Can you work these out from the model? Positions are in its coordinate system, mm. A direction names the side the tool comes from. Round coordinates to 2 decimals unless told otherwise and drop trailing zeros. Loops run counter-clockwise (first coordinate to the right, second up) from the corner with the lowest first, then second, coordinate; pieces in that order, holes last. Notation, with made-up numbers: M -34,0.25 L -27,0.25 A22 cw -27,27.25 Z; hole C 61.5,74.25 d5. An arc over 180 degrees is marked long. Answer as CSV lines item,"result".
from build123d import *

# Parameters (mm, degrees)
SKETCH1_R                                 = 21.166666667
BOSS_EXTRUDE1_DEPTH                       = 12.7
CUT_EXTRUDE_DCLTBC_DEPTH                  = 13.7
FILLET_TIP_DCLTBC_R                       = 0.376401082
FILLET_ROOT_DCLTBC_R                      = 0.752802164
CIRPATTERN_DCLTBC_COUNT                   = 18
FILLET_TIP_DCLTBC_OF_CIRPATTERN_DCLTBC_R  = 0.376401082
FILLET_ROOT_DCLTBC_OF_CIRPATTERN_DCLTBC_R = 0.752802164
SKETCH4_R                                 = 3.556
CUT_EXTRUDE2_DEPTH                        = 13.7000001
SKETCH5_R                                 = 1
CUT_EXTRUDE3_DEPTH                        = 13.7000001
BOSS_EXTRUDE3_DEPTH                       = 12.7
SKETCH9_R                                 = 1.778
CUT_EXTRUDE4_DEPTH                        = 101.6
SKETCH10_R                                = 2.75
CUT_EXTRUDE5_DEPTH                        = 7.7
CUT_EXTRUDE6_DEPTH                        = 13.7000001
CIRPATTERN1_COUNT                         = 30
CIRPATTERN1_ANGLE                         = 75
SKETCH12_W                                = 54.92757211
SKETCH12_H                                = 48.855993121
CUT_EXTRUDE7_DEPTH                        = 13.7000001


with BuildPart() as part:
    # Sketch1 → Boss-Extrude1 (new body)
    with BuildSketch(Plane.XY):
        Circle(SKETCH1_R)
    extrude(amount=BOSS_EXTRUDE1_DEPTH)

    # DCLTBC → Cut-Extrude-DCLTBC (cut, through all)
    with BuildSketch(Plane.XY):
        with BuildLine():
            Line((-0.988599485, 17.23683661), (-0.939299003, 16.37725256))
            ThreePointArc((-0.939299003, 16.37725256), (0, 16.404166667), (0.939299003, 16.37725256))
            Line((0.939299003, 16.37725256), (0.988599485, 17.23683661))
            add(Edge.make_bspline(
                [(0.988599485, 17.23683661), (0.989063314, 17.24324115), (0.990661792, 17.261181979), (0.994858273, 17.295004515), (1.003369641, 17.350013815), (1.016655031, 17.419804647), (1.036619493, 17.509601098), (1.063718234, 17.614795353), (1.097234262, 17.729707804), (1.137709634, 17.85389969), (1.181621422, 17.977005275), (1.228695452, 18.099012466), (1.278527467, 18.219794849), (1.342341331, 18.365146152), (1.42364652, 18.538069209), (1.525589195, 18.738036686), (1.649316002, 18.962165854), (1.783980218, 19.187521629), (1.923498112, 19.406676656), (2.072405817, 19.624910262), (2.222105415, 19.833784741), (2.385586794, 20.047220122), (2.540566559, 20.242458208), (2.722891612, 20.457068476), (2.872582231, 20.629074977), (3.034353491, 20.803165616), (3.114136758, 20.887359483), (3.155350355, 20.930158669)],
                knots=[0, 0, 0, 0, 0, 0.005376749, 0.015083688, 0.02853182, 0.04661014, 0.064854849, 0.092110525, 0.119476176, 0.146842496, 0.174208854, 0.201574956, 0.228941013, 0.256307345, 0.307035032, 0.361767352, 0.416499661, 0.471231937, 0.525964282, 0.580696616, 0.635428982, 0.690161387, 0.744893688, 0.799626082, 0.854358408, 0.909090915, 0.909090915, 0.909090915, 0.909090915, 0.909090915], degree=4))
            ThreePointArc((3.155350355, 20.930158669), (0, 21.166666667), (-3.155350355, 20.930158669))
            add(Edge.make_bspline(
                [(-0.988599485, 17.23683661), (-0.989063314, 17.24324115), (-0.990661792, 17.261181979), (-0.994858273, 17.295004515), (-1.003369641, 17.350013815), (-1.016655031, 17.419804647), (-1.036619493, 17.509601098), (-1.063718234, 17.614795353), (-1.097234262, 17.729707804), (-1.137709634, 17.85389969), (-1.181621422, 17.977005275), (-1.228695452, 18.099012466), (-1.278527467, 18.219794849), (-1.342341331, 18.365146152), (-1.42364652, 18.538069209), (-1.525589195, 18.738036686), (-1.649316002, 18.962165854), (-1.783980218, 19.187521629), (-1.923498112, 19.406676656), (-2.072405817, 19.624910262), (-2.222105415, 19.833784741), (-2.385586794, 20.047220122), (-2.540566559, 20.242458208), (-2.722891612, 20.457068476), (-2.872582231, 20.629074977), (-3.034353491, 20.803165616), (-3.114136758, 20.887359483), (-3.155350355, 20.930158669)],
                knots=[0, 0, 0, 0, 0, 0.005376749, 0.015083688, 0.02853182, 0.04661014, 0.064854849, 0.092110525, 0.119476176, 0.146842496, 0.174208854, 0.201574956, 0.228941013, 0.256307345, 0.307035032, 0.361767352, 0.416499661, 0.471231937, 0.525964282, 0.580696616, 0.635428982, 0.690161387, 0.744893688, 0.799626082, 0.854358408, 0.909090915, 0.909090915, 0.909090915, 0.909090915, 0.909090915], degree=4))
        make_face()
    cut_extrude_dcltbc = extrude(amount=CUT_EXTRUDE_DCLTBC_DEPTH, mode=Mode.SUBTRACT)

    # Fillet-Tip-DCLTBC
    fillet_tip_dcltbc_edges = [part.edges().sort_by_distance(p)[0] for p in [
        (3.155350355, 20.930158669, 6.35),
        (-3.155350355, 20.930158669, 6.35),
    ]]
    fillet(fillet_tip_dcltbc_edges, radius=FILLET_TIP_DCLTBC_R)

    # Fillet-Root-DCLTBC
    fillet_root_dcltbc_edges = [part.edges().sort_by_distance(p)[0] for p in [
        (0.939299003, 16.37725256, 6.35),
        (-0.939299003, 16.37725256, 6.35),
    ]]
    fillet(fillet_root_dcltbc_edges, radius=FILLET_ROOT_DCLTBC_R)

    # CirPattern-DCLTBC: Cut-Extrude-DCLTBC ×18 about axis
    cirpattern_dcltbc_axis = Axis((0, 0, 12.7), (0, 0, 1))
    for i in range(1, CIRPATTERN_DCLTBC_COUNT):
        add(cut_extrude_dcltbc.rotate(cirpattern_dcltbc_axis, i * 360 / CIRPATTERN_DCLTBC_COUNT), mode=Mode.SUBTRACT)

    # Fillet-Tip-DCLTBC of CirPattern-DCLTBC
    fillet_tip_dcltbc_of_cirpattern_dcltbc_edges = [part.edges().sort_by_distance(p)[0] for p in [
        (-4.193476424, 20.747109034, 6.35),
        (-10.123595312, 18.588722273, 6.35),
        (-11.036508056, 18.061651854, 6.35),
        (-15.870785267, 14.00521163, 6.35),
        (-16.548373935, 13.1976929, 6.35),
        (-19.70372429, 7.73246577, 6.35),
        (-20.06426169, 6.741897404, 6.35),
        (-21.160103368, 0.527070418, 6.35),
        (-21.160103368, -0.527070418, 6.35),
        (-20.06426169, -6.741897404, 6.35),
        (-19.70372429, -7.73246577, 6.35),
        (-16.548373935, -13.1976929, 6.35),
        (-15.870785267, -14.00521163, 6.35),
        (-11.036508056, -18.061651854, 6.35),
        (-10.123595312, -18.588722273, 6.35),
        (-4.193476424, -20.747109034, 6.35),
        (-3.155350355, -20.930158669, 6.35),
        (3.155350355, -20.930158669, 6.35),
        (4.193476424, -20.747109034, 6.35),
        (10.123595312, -18.588722273, 6.35),
        (11.036508056, -18.061651854, 6.35),
        (15.870785267, -14.00521163, 6.35),
        (16.548373935, -13.1976929, 6.35),
        (19.70372429, -7.73246577, 6.35),
        (20.06426169, -6.741897404, 6.35),
        (21.160103368, -0.527070418, 6.35),
        (21.160103368, 0.527070418, 6.35),
        (20.06426169, 6.741897404, 6.35),
        (19.70372429, 7.73246577, 6.35),
        (16.548373935, 13.1976929, 6.35),
        (15.870785267, 14.00521163, 6.35),
        (11.036508056, 18.061651854, 6.35),
        (10.123595312, 18.588722273, 6.35),
        (4.193476424, 20.747109034, 6.35),
    ]]
    fillet(fillet_tip_dcltbc_of_cirpattern_dcltbc_edges, radius=FILLET_TIP_DCLTBC_OF_CIRPATTERN_DCLTBC_R)

    # Fillet-Root-DCLTBC of CirPattern-DCLTBC
    fillet_root_dcltbc_of_cirpattern_dcltbc_edges = [part.edges().sort_by_distance(p)[0] for p in [
        (-4.718697926, 15.710842559, 6.35),
        (-6.48400261, 15.0683242, 6.35),
        (-9.807550244, 13.149473078, 6.35),
        (-11.246639808, 11.941933556, 6.35),
        (-13.71346726, 9.002083078, 6.35),
        (-14.652766263, 7.375169482, 6.35),
        (-15.965337734, 3.768909003, 6.35),
        (-16.291552854, 1.918851122, 6.35),
        (-16.291552854, -1.918851122, 6.35),
        (-15.965337734, -3.768909003, 6.35),
        (-14.652766263, -7.375169482, 6.35),
        (-13.71346726, -9.002083078, 6.35),
        (-11.246639808, -11.941933556, 6.35),
        (-9.807550244, -13.149473078, 6.35),
        (-6.48400261, -15.0683242, 6.35),
        (-4.718697926, -15.710842559, 6.35),
        (-0.939299003, -16.37725256, 6.35),
        (0.939299003, -16.37725256, 6.35),
        (4.718697926, -15.710842559, 6.35),
        (6.48400261, -15.0683242, 6.35),
        (9.807550244, -13.149473078, 6.35),
        (11.246639808, -11.941933556, 6.35),
        (13.71346726, -9.002083078, 6.35),
        (14.652766263, -7.375169482, 6.35),
        (15.965337734, -3.768909003, 6.35),
        (16.291552854, -1.918851122, 6.35),
        (16.291552854, 1.918851122, 6.35),
        (15.965337734, 3.768909003, 6.35),
        (14.652766263, 7.375169482, 6.35),
        (13.71346726, 9.002083078, 6.35),
        (11.246639808, 11.941933556, 6.35),
        (9.807550244, 13.149473078, 6.35),
        (6.48400261, 15.0683242, 6.35),
        (4.718697926, 15.710842559, 6.35),
    ]]
    fillet(fillet_root_dcltbc_of_cirpattern_dcltbc_edges, radius=FILLET_ROOT_DCLTBC_OF_CIRPATTERN_DCLTBC_R)

    # Sketch4 → Cut-Extrude2 (cut, through all)
    with BuildSketch(Plane.XY.offset(12.7)):
        Circle(SKETCH4_R)
    extrude(amount=-CUT_EXTRUDE2_DEPTH, mode=Mode.SUBTRACT)

    # Sketch5 → Cut-Extrude3 (cut, through all)
    with BuildSketch(Plane.XY.offset(12.7)):
        with Locations((-7, 0)):
            Circle(SKETCH5_R)
        with Locations((0, 7)):
            Circle(SKETCH5_R)
        with Locations((7, 0)):
            Circle(SKETCH5_R)
        with Locations((0, -7)):
            Circle(SKETCH5_R)
    extrude(amount=-CUT_EXTRUDE3_DEPTH, mode=Mode.SUBTRACT)

    # Sketch7 → Boss-Extrude3 (add, through all)
    with BuildSketch(Plane.XY.offset(12.7)):
        with BuildLine():
            Line((6.35, -14.113720517), (6.35, -26.813720517))
            ThreePointArc((6.35, -26.813720517), (16.563553869, -62.204697552), (3.547653041, -96.663720517))
            Line((3.547653041, -96.663720517), (-15.629346959, -96.663720517))
            Line((-15.629346959, -96.663720517), (-2.2365023, -91.788432197))
            ThreePointArc((-2.2365023, -91.788432197), (9.041883703, -59.131392983), (-3.175, -26.813720517))
            Line((-3.175, -26.813720517), (-3.175, -14.113720517))
            Line((-3.175, -14.113720517), (6.35, -14.113720517))
        make_face()
    extrude(amount=-BOSS_EXTRUDE3_DEPTH)

    # Sketch9 → Cut-Extrude4 (cut)
    with BuildSketch(Plane.XY.offset(12.7)):
        with Locations((5.222816577, -31.033083261)):
            Circle(SKETCH9_R)
        with Locations((9.993601717, -78.846696124)):
            Circle(SKETCH9_R)
    extrude(amount=-CUT_EXTRUDE4_DEPTH, mode=Mode.SUBTRACT)

    # Sketch10 → Cut-Extrude5 (cut)
    with BuildSketch(Plane.XY.offset(12.7)):
        with Locations((-7, 0)):
            Circle(SKETCH10_R)
        with Locations((0, -7)):
            Circle(SKETCH10_R)
        with Locations((7, 0)):
            Circle(SKETCH10_R)
        with Locations((0, 7)):
            Circle(SKETCH10_R)
    extrude(amount=-CUT_EXTRUDE5_DEPTH, mode=Mode.SUBTRACT)

    # Sketch11 → Cut-Extrude6 (cut, through all)
    with BuildSketch(Plane.XY.offset(12.7)):
        with BuildLine():
            Line((-2.2365023, -91.788432197), (-0.9665023, -91.788432197))
            Line((-0.9665023, -91.788432197), (-1.271582988, -90.555620056))
            ThreePointArc((-1.271582988, -90.555620056), (-1.749293325, -91.175743408), (-2.2365023, -91.788432197))
        make_face()
    cut_extrude6 = extrude(amount=-CUT_EXTRUDE6_DEPTH, mode=Mode.SUBTRACT)

    # CirPattern1: Cut-Extrude6 ×30 about axis
    cirpattern1_axis = Axis((-41.752817912, -59.865073971, 0), (0, 0, 1))
    for i in range(1, CIRPATTERN1_COUNT):
        add(cut_extrude6.rotate(cirpattern1_axis, i * CIRPATTERN1_ANGLE / (CIRPATTERN1_COUNT - 1)), mode=Mode.SUBTRACT)

    # Sketch12 → Cut-Extrude7 (cut, through all)
    with BuildSketch(Plane.XY.offset(12.7)):
        with Locations((1.598076801, -2.385723956)):
            Rectangle(SKETCH12_W, SKETCH12_H)
    extrude(amount=-CUT_EXTRUDE7_DEPTH, mode=Mode.SUBTRACT)


solid = part.part
Item 1: If we section it at A-A on x = 13.5: Write out the boundary of the cut face in (y, z).
Output:
outline,"M -78.66,0 L -41.07,0 L -41.07,12.7 L -78.66,12.7 Z"
Item 2: On a 3-axis mill with a long thin cutter (end or side, diameter ignored), from which of +Z, -Z, +X, -X, +Y, -Y can I reach the whole of each face in a straight line? I mean faces 4 (the face through (4.84, -32.77, 6.44)), 5 (the face through (-0.211, -89.945, 6.439)). Say none if no direction works.
Output:
face 4,"+Z, -Z"
face 5,"+Z, -Z, -X"
Item 3: If we section it at C-C on x = -9: Write out the boundary of the cut face in (y, z).
Output:
outline,"M -96.66,0 L -94.25,0 L -94.25,12.7 L -96.66,12.7 Z"
Item 4: Will these pins go through, and if not, where does the flat tip stop? pin 1 (4 mm diameter, centred on y = -73.5, z = 5, fed in from +X); pin 2 (8 mm diameter, centred on x = 4, y = -61, fed in from -Z); pin 3 (3 mm diameter, centred on y = -39.5, z = 7.5, fed in from +X); pin 4 (4 mm diameter, centred on y = -68.5, z = 3, fed in from +X).
Output:
pin 1,"stops at x = 15.44"
pin 2,"passes through"
pin 3,"stops at x = 13.48"
pin 4,"stops at x = 16.23"
Item 5: We'd pull the mould along Y, two halves only. Please class faces 1 (the face through (16.582, -61.68, 6.439)), 2 (the face through (7.39, -45.13, 6.44)), 3 (the face through (10, -62, 0)): released by +Y, released by -Y, zero draft, split by the parting line, or undercut.
Output:
face 1,"split by the parting line"
face 2,"undercut"
face 3,"zero draft"
Item 6: If we section it at B-B on z = 2.5: State how many separate pieces and enclosed holes the cut face has, then the cut area to 3 significant figures.
Output:
separate pieces,"1"
enclosed holes,"2"
area,"553 mm2"
Item 7: If I drill on line 1 along X through (y, z) = (-59.5, 8); line 2 along X through (y, z) = (-47, 3.5); line 3 along Y through (x, z) = (-13, 6.5), over which ranges is the centre line in solid material (lowest first)? Write a range as from..to.
Output:
line 1,"x = 9.66..16.61"
line 2,"x = 7.39..15.17"
line 3,"y = -96.66..-95.71"
